from build123d import *

# Parameters (mm, degrees)
SKETCH_1_R      = 1.7
EXTRUDE_1_DEPTH = 0.5


with BuildPart() as part:
    # Эскиз1 → Бобышка-Вытянуть1 (new body)
    with BuildSketch(Plane(origin=(0, 0, 0), x_dir=(1, 0, 0), z_dir=(0, 1, 0))):
        with BuildLine():
            Line((-40.771031168, -46.911249121), (41.728968832, -46.911249121))
            ThreePointArc((41.728968832, -46.911249121), (42.93105036, -46.413330649), (43.428968832, -45.211249121))
            Line((43.428968832, -45.211249121), (43.428968832, 44.788750879))
            ThreePointArc((43.428968832, 44.788750879), (42.93105036, 45.990832407), (41.728968832, 46.488750879))
            Line((41.728968832, 46.488750879), (-40.771031168, 46.488750879))
            ThreePointArc((-40.771031168, 46.488750879), (-41.973112696, 45.990832407), (-42.471031168, 44.788750879))
            Line((-42.471031168, 44.788750879), (-42.471031168, -45.211249121))
            ThreePointArc((-42.471031168, -45.211249121), (-41.973112696, -46.413330649), (-40.771031168, -46.911249121))
        make_face()
        with Locations((-39.371031168, -0.211249121)):
            Circle(SKETCH_1_R, mode=Mode.SUBTRACT)
        with Locations((-39.371031168, -43.811249121)):
            Circle(SKETCH_1_R, mode=Mode.SUBTRACT)
        with Locations((0.478968832, -43.811249121)):
            Circle(SKETCH_1_R, mode=Mode.SUBTRACT)
        with Locations((40.328968832, -43.811249121)):
            Circle(SKETCH_1_R, mode=Mode.SUBTRACT)
        with Locations((40.328968832, -0.211249121)):
            Circle(SKETCH_1_R, mode=Mode.SUBTRACT)
        with Locations((40.328968832, 43.388750879)):
            Circle(SKETCH_1_R, mode=Mode.SUBTRACT)
        with Locations((0.478968832, 43.388750879)):
            Circle(SKETCH_1_R, mode=Mode.SUBTRACT)
        with Locations((-39.371031168, 43.388750879)):
            Circle(SKETCH_1_R, mode=Mode.SUBTRACT)
        with BuildLine():
            Line((-39.371031168, 39.987280609), (-39.371031168, 2.888750879))
            ThreePointArc((-39.371031168, 2.888750879), (-36.271031168, -0.211249121), (-39.371031168, -3.311249121))
            Line((-39.371031168, -3.311249121), (-39.371031168, -40.40977885))
            ThreePointArc((-39.371031168, -40.40977885), (-36.965828473, -41.406046427), (-35.969560897, -43.811249121))
            Line((-35.969560897, -43.811249121), (-2.621031168, -43.811249121))
            ThreePointArc((-2.621031168, -43.811249121), (0.478968832, -40.711249121), (3.578968832, -43.811249121))
            Line((3.578968832, -43.811249121), (36.927498562, -43.811249121))
            ThreePointArc((36.927498562, -43.811249121), (37.923766138, -41.406046427), (40.328968832, -40.40977885))
            Line((40.328968832, -40.40977885), (40.328968832, -3.311249121))
            ThreePointArc((40.328968832, -3.311249121), (37.228968832, -0.211249121), (40.328968832, 2.888750879))
            Line((40.328968832, 2.888750879), (40.328968832, 39.987280609))
            ThreePointArc((40.328968832, 39.987280609), (37.923766138, 40.983548185), (36.927498562, 43.388750879))
            Line((36.927498562, 43.388750879), (3.578968832, 43.388750879))
            ThreePointArc((3.578968832, 43.388750879), (0.478968832, 40.288750879), (-2.621031168, 43.388750879))
            Line((-2.621031168, 43.388750879), (-35.969560897, 43.388750879))
            ThreePointArc((-35.969560897, 43.388750879), (-36.965828473, 40.983548185), (-39.371031168, 39.987280609))
        make_face(mode=Mode.SUBTRACT)
    extrude(amount=EXTRUDE_1_DEPTH)


solid = part.part
The listing builds one solid part. Answer for the finished solid, in the listing's coordinates (mm). A direction names the side the tool comes from. Coordinates: 2 decimals unless noted, no trailing zeros. Order: outer loops, then holes, each group sorted by start corner. A loop starts at its lowest first (then second) coordinate and runs counter-clockwise, first axis right, second up. Notation, with made-up numbers: M 73,-34.5 L 100,-34.5 A19 ccw 100,-9.5 Z; hole C 52,41 d11. An arc over 180 degrees is marked long. Use CSV: the item, a comma, the result in double quotes.
Q1. Section C-C (y = 0.1) is taken. Give the number of separate pieces and of enclosed holes in the cut face, then the cut area to 3 significant figures.
Here are the results:
separate pieces,"1"
enclosed holes,"9"
area,"1,090 mm2"
Q2. Section B-B (z = -36) is taken. Determine the outline of the cut face in (x, y).
Here are the results:
outline,"M -42.47,0 L -39.37,0 L -39.37,0.5 L -42.47,0.5 Z; M 40.33,0 L 43.43,0 L 43.43,0.5 L 40.33,0.5 Z"
Q3. A tool of negligible diameter and unlimited length cuts with its end or side. For faces 1 (the flat face through (0.3, 0, -41.5)), 2 (the cylindrical face through (37.9, 0.25, 41.43)), from which of +Z, -Z, +X, -X, +Y, -Y can it reach the whole face along a straight path? Write none if from no direction.
Here are the results:
face 1,"+Z, -Z, +X, -X, -Y"
face 2,"+Y, -Y"
Q4. Straight lines are drawn through the part: L1, parallel to X at y = 0.45, z = -28; L2, parallel to Z at x = -8.5, y = 0.2; L3, parallel to X at y = 0.3, z = -41. For each, find the intervals that lie inside material, in ascending order.
Here are the results:
L1,"-42.47 to -39.37, 40.33 to 43.43"
L2,"-46.49 to -43.39, 43.81 to 46.91"
L3,"-42.47 to -36.95, -1.5 to 2.45, 37.91 to 43.43"
Q5. Given pin 1 Ø5 at (x, z) = (34.5, -1.5) entering from +Y, flat-ended and moving along its own axis, determine where the tip first touches the part or whether it passes through.
Here are the results:
pin 1,"through"
Q6. Section A-A (x = -21) is taken. Determine the outline of the cut face in (y, z), then the cut area to 3 significant figures.
Here are the results:
outline,"M 0,-46.49 L 0.5,-46.49 L 0.5,-43.39 L 0,-43.39 Z; M 0,43.81 L 0.5,43.81 L 0.5,46.91 L 0,46.91 Z"
area,"3.10 mm2"
Q7. Determine the mould class of faces 3 (the cylindrical face through (41.243, 0.246, 42.378)), 4 (the flat face through (0.3, 0.5, -41.5)) for opening direction Z: pulls with the +Z half, pulls with the -Z half, needs draft (parallel to the pull), parting line crosses it, or undercut.
Here are the results:
face 3,"undercut"
face 4,"needs draft"
